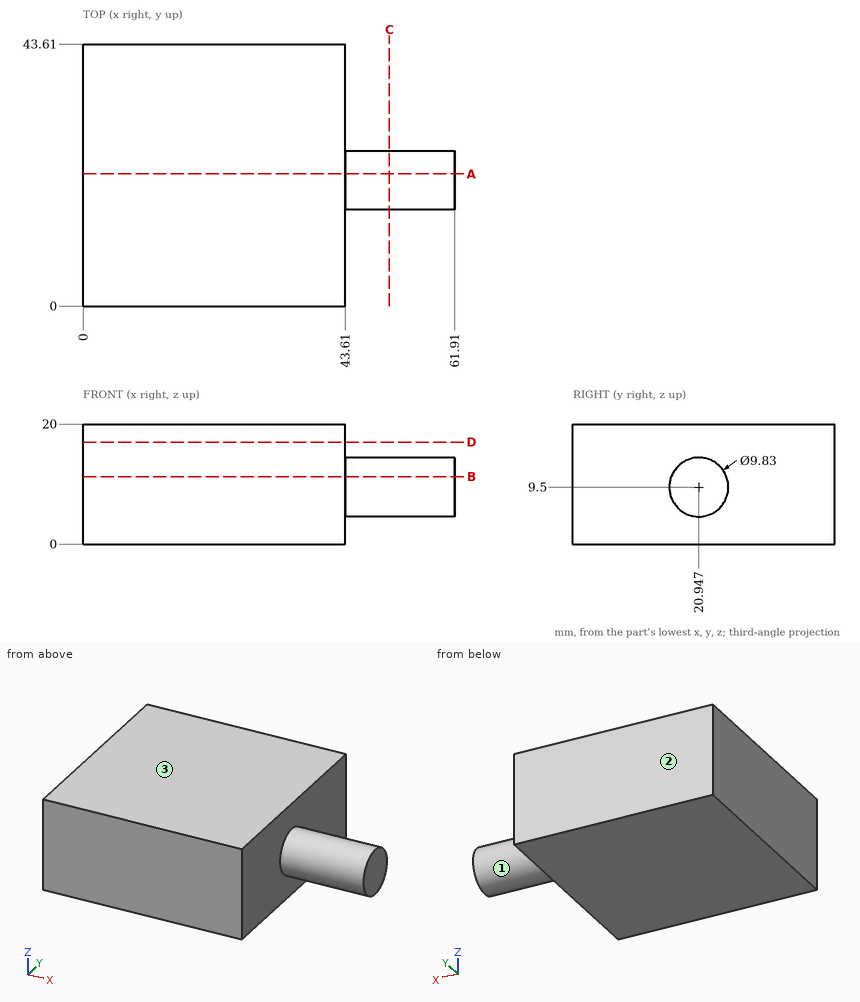
Print and shaded views of the part. All mm, measured from the part's lowest x, y and z. Coordinates: 2 decimals unless noted, no trailing zeros. Order: outer loops, then holes, each group sorted by start corner. A loop starts at its lowest first (then second) coordinate and runs counter-clockwise, first axis right, second up. Notation, with made-up numbers: (-17.75, -7.75) -> (-13.75, -7.75) arc R18 ccw to (-13.75, 7.25) -> close; hole circle Ø8 at (6, -31.75). An arc over 180 degrees is marked (long way). Use one line per item in the form item = value. Start each with the question number.
1) Band-saw the part on B-B on z = 11.25. Give the cut face in (x, y), then the cut area to 3 significant figures.
2) Band-saw the part on C-C on x = 51. Give the cut face in (y, z) (1 decimal), then the cut area to 3 significant figures.
3) Pull direction Y, two halves, no side cores. Call the marked faces 1, 2 and 3: +Y half, -Y half, draft (parallel to the pull), parting line (faces both ways), or undercut.
4) Drop flat-ended pins along their axis: pin 1 (8 mm diameter, centred on x = 50.5, y = 21, fed in from -Z) (1 decimal); pin 2 (2 mm diameter, centred on y = 33, z = 3.5, fed in from +X); pin 3 (3 mm diameter, centred on x = 48, z = 11.5, fed in from -Y). Give the stop position or say it passes through.
5) Band-saw the part on D-D on z = 17. Give the cut face in (x, y), then the cut area to 3 significant figures.
6) Band-saw the part on A-A on y = 22. Give the cut face in (x, z), then the cut area to 3 significant figures.
7) Drill centre lines: L1, parallel to X at y = 30, z = 17.5; L2, parallel to Y at x = 51, z = 9.5; L3, parallel to Z at x = 52, y = 23 (1 decimal). Where is each one in solid material? Low to high. Write a range as [from, to].
Entries:
q1.outline = (0, 0) -> (43.61, 0) -> (43.61, 16.35) -> (61.91, 16.35) -> (61.91, 25.54) -> (43.61, 25.54) -> (43.61, 43.61) -> (0, 43.61) -> close
q1.area = 2,070 mm2
q2.outline = circle Ø9.8 at (20.9, 9.5)
q2.area = 75.9 mm2
q3.face_1 = parting line
q3.face_2 = +Y half
q3.face_3 = draft
q4.pin_1 = 4.6
q4.pin_2 = 43.61
q4.pin_3 = 16.06
q5.outline = (0, 0) -> (43.61, 0) -> (43.61, 43.61) -> (0, 43.61) -> close
q5.area = 1,900 mm2
q6.outline = (0, 0) -> (43.61, 0) -> (43.61, 4.7) -> (61.91, 4.7) -> (61.91, 14.3) -> (43.61, 14.3) -> (43.61, 20) -> (0, 20) -> close
q6.area = 1,050 mm2
q7.L1 = [0, 43.61]
q7.L2 = [16.03, 25.86]
q7.L3 = [5, 14]
